Can you work these out from the drawing? Everything is in mm from the part's minimum corner. A direction names the side the tool comes from. Give positions to 0.01 mm unless a question says otherwise; leave off trailing zeros. Loops run counter-clockwise (first coordinate to the right, second up) from the corner with the lowest first, then second, coordinate; pieces in that order, holes last. Notation, with made-up numbers: (59.25, 17) - (103.25, 17) arc R16 cw to (103.25, 46) - close; hole circle Ø6 at (29.25, 34.5). An arc over 180 degrees is marked (long way). Answer in a Markdown table with one row per item.
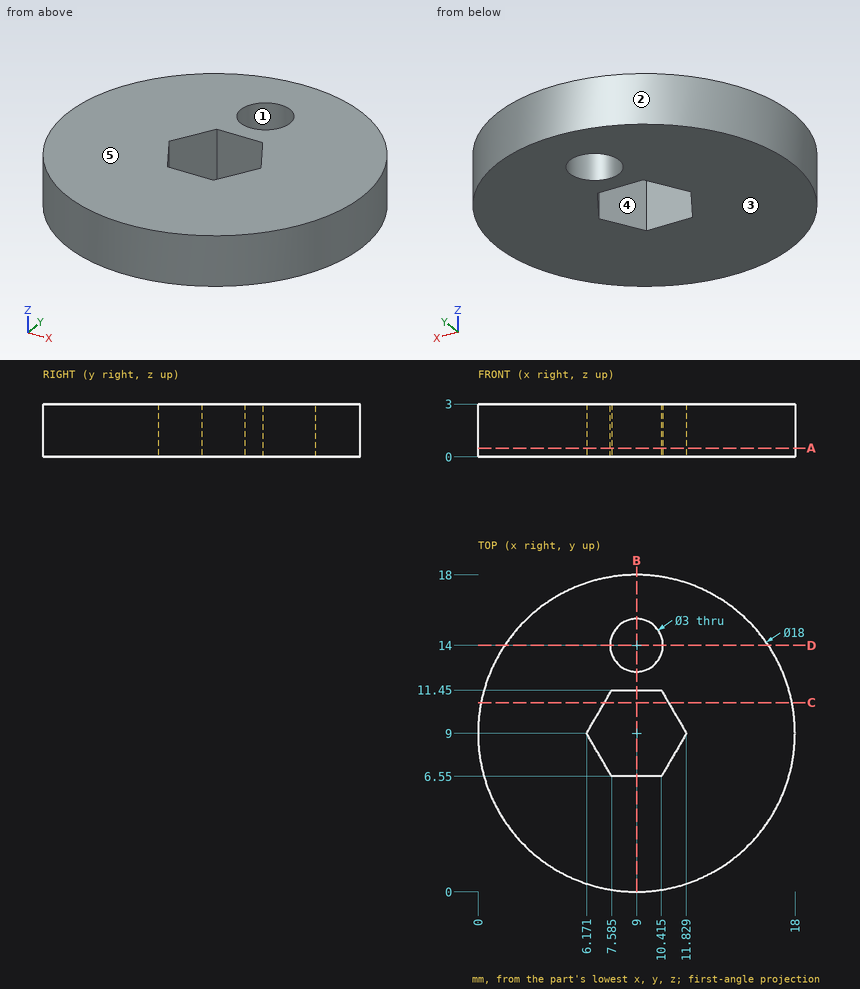
Q1. Imagine slicing it at B-B, the plane x = 9. Write out the boundary of the cut face in (y, z).
Checked values:
| item | result |
|---|---|
| outline | (0, 0) - (6.55, 0) - (6.55, 3) - (0, 3) - close; (11.45, 0) - (12.5, 0) - (12.5, 3) - (11.45, 3) - close; (15.5, 0) - (18, 0) - (18, 3) - (15.5, 3) - close |
Q2. If we mould it in two halves opening along Y, with no side actions, what happens to the marked faces 1, 2 and 3? For each: released by +Y, released by -Y, zero draft, split by the parting line, or undercut.
Checked values:
| item | result |
|---|---|
| face 1 | undercut |
| face 2 | split by the parting line |
| face 3 | zero draft |
Q3. If I drill on line 1 (Y direction, x = 9, z = 1.55); line 2 (Y direction, x = 4.5, z = 1.25) (1 decimal); line 3 (X direction, y = 3.25, z = 0.7) (1 decimal), over which ranges is the centre line in solid material (lowest first)? Write a range as [from, to].
Checked values:
| item | result |
|---|---|
| line 1 | y = [0, 6.55], [11.45, 12.5], [15.5, 18] |
| line 2 | y = [1.2, 16.8] |
| line 3 | x = [2.1, 15.9] |
Q4. Imagine slicing it at D-D, the plane y = 14. Write out the boundary of the cut face in (x, z).
Checked values:
| item | result |
|---|---|
| outline | (1.52, 0) - (7.5, 0) - (7.5, 3) - (1.52, 3) - close; (10.5, 0) - (16.48, 0) - (16.48, 3) - (10.5, 3) - close |
Q5. Imagine slicing it at C-C, the plane y = 10.75. Write out the boundary of the cut face in (x, z).
Checked values:
| item | result |
|---|---|
| outline | (0.17, 0) - (7.18, 0) - (7.18, 3) - (0.17, 3) - close; (10.82, 0) - (17.83, 0) - (17.83, 3) - (10.82, 3) - close |
Q6. Imagine slicing it at A-A, the plane z = 0.5. Count the separate pieces of the cut face and the enclosed holes in it, and give its area (3 significant figures).
Checked values:
| item | result |
|---|---|
| separate pieces | 1 |
| enclosed holes | 2 |
| area | 227 mm² |
Q7. For pin 1 (1.5 mm diameter, centred on y = 11, z = 1, fed in from +X); pin 2 (1 mm diameter, centred on y = 8, z = 1.5, fed in from +X); pin 3 (1.4 mm diameter, centred on x = 9.5, z = 2, fed in from -Y), each with a flat end and sliding along its axis, tell me the tip position at first contact or that it passes through.
Checked values:
| item | result |
|---|---|
| pin 1 | stops at x = 17.91 |
| pin 2 | stops at x = 17.99 |
| pin 3 | stops at y = 0 |
Q8. On a 3-axis mill with a long thin cutter (end or side, diameter ignored), from which of +Z, -Z, +X, -X, +Y, -Y can I reach the whole of each face in a straight line? I mean the marked faces 4 and 5. Say none if no direction works.
Checked values:
| item | result |
|---|---|
| face 4 | +Z, -Z |
| face 5 | +Z, +X, -X, +Y, -Y |
